```python
from build123d import *

# Parameters (mm, degrees)
F0_W     = 110
F0_H     = 90
F0_R     = 11.15
F1_DEPTH = 3
F2_R     = 2.5
F3_DEPTH = 3
F4_R     = 5


with BuildPart() as f1:
    # F0 (on Front) → F1 (new body)
    with BuildSketch(Plane.XZ):
        Rectangle(F0_W, F0_H)
        with Locations((-27.5, -17.5)):
            Circle(F0_R, mode=Mode.SUBTRACT)
        with Locations((27.5, -17.5)):
            Circle(F0_R, mode=Mode.SUBTRACT)
        with Locations((-27.5, 17.5)):
            Circle(F0_R, mode=Mode.SUBTRACT)
        with Locations((27.5, 17.5)):
            Circle(F0_R, mode=Mode.SUBTRACT)
    extrude(amount=F1_DEPTH)

    # F2 (on face) → F3 (cut, through all)
    with BuildSketch(Plane.XZ.offset(3)):
        with Locations((-50, 40)):
            Circle(F2_R)
        with Locations((50, 40)):
            Circle(F2_R)
        with Locations((50, -40)):
            Circle(F2_R)
        with Locations((-50, -40)):
            Circle(F2_R)
    extrude(amount=-F3_DEPTH, mode=Mode.SUBTRACT)

    # F4
    f4_edges = [f1.edges().sort_by_distance(p)[0] for p in [
        (55, -1.5, 45),
        (-55, -1.5, 45),
        (55, -1.5, -45),
        (-55, -1.5, -45),
    ]]
    fillet(f4_edges, radius=F4_R)


solid = f1.part
```
CAD build for the part. Positions are in the model's coordinates, mm. Coordinates: 2 decimals unless noted, no trailing zeros. Order: outer loops, then holes, each group sorted by start corner. A loop starts at its lowest first (then second) coordinate and runs counter-clockwise, first axis right, second up. Notation, with made-up numbers: M 52,17.5 L 77,17.5 A17 ccw 77,31.5 Z; hole C 84.25,34.25 d5. An arc over 180 degrees is marked long. Write each question's results on one line, items separated by ' | '. Start each with the question number.
Q1. Cut at B-B (x = -27.5). List the corners of the cut face in (y, z).
Q2. Cut at C-C (y = -2). Count the separate pieces of the cut face and the enclosed holes in it, then the cut area to 3 significant figures.
Q3. Flat gauge pins, fed straight in: P1, Ø8, axis at x = -28, z = -35.5, coming from the +Y side; P2, Ø4.5, axis at x = 50, z = -40, coming from the -Y side. Where does each tip first touch, or does it go through?
Q4. Cut at A-A (z = -17.5). List the corners of the cut face in (x, y), then the cut area to 3 significant figures.
Q5. Drill centre lines: probe 1 along X at (y, z) = (-1.55, 18); probe 2 along Z at (x, y) = (-28, -1.8); probe 3 along Z at (x, y) = (-50, -0.15). Where is each one in solid material? Low to high. Write a range as from..to.
Q6. Pull direction X, two halves, no side cores. Call faces 1 (the cylindrical face through (53, -2, -44)), 2 (the flat face through (-1, -3, 1)), 3 (the cylindrical face through (-47.69, -1.52, 39.04)): +X half, -X half, draft (parallel to the pull), parting line (faces both ways), or undercut.
Found:
1) outline: M -3,-45 L 0,-45 L 0,-28.65 L -3,-28.65 Z; M -3,-6.35 L 0,-6.35 L 0,6.35 L -3,6.35 Z; M -3,28.65 L 0,28.65 L 0,45 L -3,45 Z
2) separate pieces: 1 | enclosed holes: 8 | area: 8,240 mm²
3) P1: y = 0 | P2: through
4) outline: M -55,-3 L -38.65,-3 L -38.65,0 L -55,0 Z; M -16.35,-3 L 16.35,-3 L 16.35,0 L -16.35,0 Z; M 38.65,-3 L 55,-3 L 55,0 L 38.65,0 Z | area: 196 mm²
5) probe 1: -55..-38.64, -16.36..16.36, 38.64..55 | probe 2: -45..-28.64, -6.36..6.36, 28.64..45 | probe 3: -45..-42.5, -37.5..37.5, 42.5..45
6) face 1: +X half | face 2: draft | face 3: undercut
